from build123d import *

# Parameters (mm, degrees)
SKETCH_1_W      = 80
SKETCH_1_H      = 3
EXTRUDE_1_DEPTH = 5
SKETCH_3_R      = 2.5
EXTRUDE_2_DEPTH = 1.5


with BuildPart() as part:
    # 草图1 → 凸台-拉伸1 (new, symmetric)
    with BuildSketch(Plane(origin=(0, 0, 0), x_dir=(1, 0, 0), z_dir=(0, 1, 0))):
        Rectangle(SKETCH_1_W, SKETCH_1_H)
    extrude(amount=EXTRUDE_1_DEPTH, both=True)

    # 草图3 → 凸台-拉伸2 (add, symmetric)
    with BuildSketch(Plane.XY):
        with BuildLine():
            Line((-15, 5), (15, 5))
            ThreePointArc((15, 5), (0, 20), (-15, 5))
        make_face()
        with Locations((0, 13)):
            Circle(SKETCH_3_R, mode=Mode.SUBTRACT)
    extrude(amount=EXTRUDE_2_DEPTH, both=True)


solid = part.part
Read the model definition and answer for the solid it produces. Units are mm, in the model's axes. A direction names the side the tool comes from. Give positions to 0.01 mm unless a question says otherwise; leave off trailing zeros. Loops run counter-clockwise (first coordinate to the right, second up) from the corner with the lowest first, then second, coordinate; pieces in that order, holes last. Notation, with made-up numbers: (9.5, -12) - (57.5, -12) arc R32 cw to (57.5, 15) - close; hole circle Ø8 at (51.5, 72.5). An arc over 180 degrees is marked (long way). Answer as CSV lines item,"result". Start each with the question number.
1) Which of the six approach directions +Z, -Z, +X, -X, +Y, -Y give full straight-line access (tool end or side, diameter ignored) to faces 4 (the face through (40, 0, 0)), 5 (the face through (-28, 5, 0))?
2) Determine the mould class of faces 1 (the face through (27, 5, 0)), 2 (the face through (-0.54, 10.56, -0.02)), 3 (the face through (-1, 5, 1.5)) for opening direction Y: released by +Y, released by -Y, zero draft, split by the parting line, or undercut.
3) Find section A-A (x = 0). Write down the section's boundary in (y, z).
4) This flat-tipped pin is pushed along its axis until it touches: pin 1 Ø1.5 at (x, z) = (32.5, 0) entering from +Y. Where does it stop, or does it pass through?
5) Straight lines are drawn through the part: L1, parallel to Y at x = 0, z = -0.15; L2, parallel to Y at x = 31, z = 0.3; L3, parallel to X at y = 11.5, z = 0.3. For each, find the intervals that lie inside material, in ascending order. Write a range as from..to.
6) Find section B-B (z = 1). Write down the section's boundary in (x, y).
7) Find section C-C (y = 13). Write down the section's boundary in (x, z), then the cut area to 3 significant figures.
8) Find section D-D (x = -18). Write down the section's boundary in (y, z), then the cut area to 3 significant figures.
Findings below:
1,face 4,"+Z, -Z, +X, +Y, -Y"
1,face 5,"+Z, -Z, -X, +Y"
2,face 1,"released by +Y"
2,face 2,"undercut"
2,face 3,"zero draft"
3,outline,"(-5, -1.5) - (10.5, -1.5) - (10.5, 1.5) - (-5, 1.5) - close; (15.5, -1.5) - (20, -1.5) - (20, 1.5) - (15.5, 1.5) - close"
4,pin 1,"y = 5"
5,L1,"-5..10.5, 15.5..20"
5,L2,"-5..5"
5,L3,"-13.52..-2, 2..13.52"
6,outline,"(-40, -5) - (40, -5) - (40, 5) - (15, 5) arc R15 ccw to (-15, 5) - (-40, 5) - close; hole circle Ø5 at (0, 13)"
7,outline,"(-12.69, -1.5) - (-2.5, -1.5) - (-2.5, 1.5) - (-12.69, 1.5) - close; (2.5, -1.5) - (12.69, -1.5) - (12.69, 1.5) - (2.5, 1.5) - close"
7,area,"61.1 mm^2"
8,outline,"(-5, -1.5) - (5, -1.5) - (5, 1.5) - (-5, 1.5) - close"
8,area,"30.0 mm^2"
